The model under review builds one solid part; all positions refer to its coordinate system, in mm. A direction names the side the tool comes from. Give positions to 0.01 mm unless a question says otherwise; leave off trailing zeros. Loops run counter-clockwise (first coordinate to the right, second up) from the corner with the lowest first, then second, coordinate; pieces in that order, holes last. Notation, with made-up numbers: (29, 65) -> (63, 65) arc R31 ccw to (63, 99) -> close; hole circle Ø8 at (4.5, -3). An arc over 180 degrees is marked (long way). Write each question's results on one line, items separated by ' | '. Start each with the question number.
Q1. Wall thickness on L1, parallel to Y at x = 27, z = 59 (3 decimals); L2, parallel to X at y = -2, z = 43; L3, parallel to Y at x = 97, z = 14.5: over which ranges is each line inside the solid? List them lowest first. Write a range as [from, to].
Q2. We need section C-C (y = 0). Write out the cut boundary in (x, z) (3 decimals).
Q3. Mouldability with a two-part tool opening along Y and no side actions: class faces 1 (the face through (45, 0, 0)), 2 (the face through (43, 3.175, 32)), 3 (the face through (40, -6.35, 29)), 4 (the face through (-7.559, -5.796, 37.567)) as released by +Y, released by -Y, zero draft, split by the parting line, or undercut.
Q4. Insertion check: pin 1 Ø10 at (x, z) = (29, 59.5) entering from -Y; pin 2 Ø8 at (x, y) = (7.5, -1.5) entering from -Z; pin 3 Ø5 at (x, y) = (56.5, 8.5) entering from +Z; pin 4 Ø8 at (x, z) = (74.5, 51) entering from +Y. Each pin has a flat end and moves straight along its axis. Give the tip position at first contact, or say it passes through.
Q5. We need section D-D (z = 5). Write out the cut boundary in (x, y) (3 decimals).
Q6. Machinability: for faces 5 (the face through (100, 5, 25.4)), 6 (the face through (41, 6.35, 29)), 7 (the face through (-9, 4, 76.2)), 8 (the face through (23.699, 0, 38)), 9 (the face through (101.26, 1.91, 12.52)), which of the approach directions +Z, -Z, +X, -X, +Y, -Y give a long, thin tool a straight path to every point of the face, cutting with its end or side? Answer none if there is none.
Q7. We need section B-B (z = 21.5). Write out the cut boundary in (x, y) (3 decimals), plus the area to 3 significant figures.
Q8. We need section A-A (x = -3). Write out the cut boundary in (y, z).
from build123d import *

# Parameters (mm, degrees)
F0_R     = 9.525
F1_DEPTH = 76.2
F3_DEPTH = 19.051
F4_R     = 10.1343674416
F4_R_2   = 6.35
F5_DEPTH = 25.4
F7_DEPTH = 3.175


with BuildPart() as f1:
    # F0 (on Top) → F1 (new body)
    with BuildSketch(Plane.XY):
        with BuildLine():
            Line((87.1985226281, 6.35), (10.9985226281, 6.35))
            ThreePointArc((10.9985226281, 6.35), (-12.7, 0), (10.9985226281, -6.35))
            Line((10.9985226281, -6.35), (87.1985226281, -6.35))
            Line((87.1985226281, -6.35), (87.1985226281, 6.35))
        make_face()
        Circle(F0_R, mode=Mode.SUBTRACT)
    extrude(amount=F1_DEPTH)

    # F2 (on face) → F3 (cut, through all)
    with BuildSketch(Plane.XZ.offset(6.35)):
        with BuildLine():
            ThreePointArc((10.9985226281, 76.2), (64.8800593545, 53.8815367264), (87.1985226281, 0))
            Line((87.1985226281, 0), (87.1985226281, 76.2))
            Line((87.1985226281, 76.2), (10.9985226281, 76.2))
        make_face()
    extrude(amount=-F3_DEPTH, mode=Mode.SUBTRACT)

    # F4 (on Top) → F5 (join)
    with BuildSketch(Plane.XY):
        with Locations((95.2044725418, 0)):
            Circle(F4_R)
        with Locations((95.2044725418, 0)):
            Circle(F4_R_2, mode=Mode.SUBTRACT)
    extrude(amount=F5_DEPTH)

    # F6 (on Front) → F7 (cut, symmetric)
    with BuildSketch(Plane.XZ):
        with BuildLine():
            Line((23.6985226281, 62.2170394667), (23.6985226281, 12.7))
            Line((23.6985226281, 12.7), (73.2155620948, 12.7))
            ThreePointArc((73.2155620948, 12.7), (55.8998032334, 44.9012806053), (23.6985226281, 62.2170394667))
        make_face()
    extrude(amount=F7_DEPTH, both=True, mode=Mode.SUBTRACT)


solid = f1.part
Output:
1) L1: [-6.35, -3.175], [3.175, 6.35] | L2: [-12.54, -9.31], [9.31, 23.7], [57.72, 73.91] | L3: [-9.97, -6.09], [6.09, 9.97]
2) outline: (-12.7, 0) -> (-9.525, 0) -> (-9.525, 76.2) -> (-12.7, 76.2) -> close; (9.525, 0) -> (88.854, 0) -> (88.854, 25.4) -> (85.07, 25.4) -> (85.07, 17.884) arc R76.2 ccw to (10.999, 76.2) -> (9.525, 76.2) -> close; (101.554, 0) -> (105.339, 0) -> (105.339, 25.4) -> (101.554, 25.4) -> close; hole (23.699, 12.7) -> (73.216, 12.7) arc R63.5 ccw to (23.699, 62.217) -> close
3) face 1: zero draft | face 2: undercut | face 3: released by -Y | face 4: undercut
4) pin 1: y = -6.35 | pin 2: z = 0 | pin 3: z = 62.05 | pin 4: through
5) outline: (10.999, -6.35) -> (87.034, -6.35) -> (87.034, -5.996) arc R10.134 ccw (long way) to (87.034, 5.996) -> (87.034, 6.35) -> (10.999, 6.35) arc R12.7 ccw (long way) to start; hole circle Ø19.05 at (0, 0); hole circle Ø12.7 at (95.204, 0)
6) face 5: +Z, +X, +Y, -Y | face 6: +Z, -Z, +Y | face 7: +Z, +X, -X, +Y, -Y | face 8: none | face 9: +Z, -Z
7) outline: (10.999, -6.35) -> (84.102, -6.35) -> (84.102, 6.35) -> (10.999, 6.35) arc R12.7 ccw (long way) to start; circle Ø20.269 at (95.204, 0); hole circle Ø19.05 at (0, 0); hole (23.699, -3.175) -> (70.748, -3.175) -> (70.748, 3.175) -> (23.699, 3.175) -> close; hole circle Ø12.7 at (95.204, 0) | area: 1,030 mm2
8) outline: (-12.34, 0) -> (-9.04, 0) -> (-9.04, 76.2) -> (-12.34, 76.2) -> close; (9.04, 0) -> (12.34, 0) -> (12.34, 76.2) -> (9.04, 76.2) -> close
